Geometry: see drawing. Coordinates: mm, zero at the bounding-box minimum. Round coordinates to 2 decimals unless told otherwise and drop trailing zeros. Order: outer loops, then holes, each group sorted by start corner. A loop starts at its lowest first (then second) coordinate and runs counter-clockwise, first axis right, second up. Notation, with made-up numbers: (76, 50.5) -> (82, 50.5) arc R22 ccw to (82, 73.5) -> close; hole circle Ø4 at (8, 51.5). An arc over 180 degrees is marked (long way). Put each result on its own line as item: value.
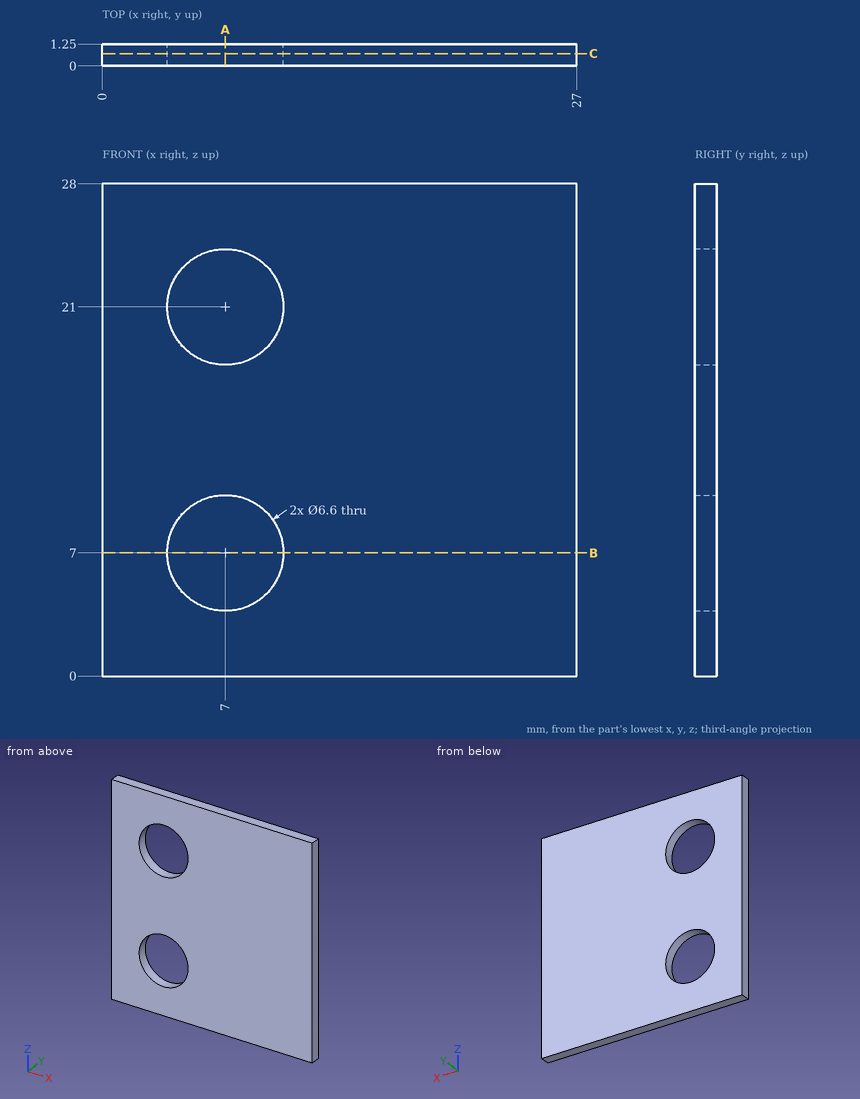
1. Cut plane A-A on x = 7. Return loops of the section in (y, z), and give its area (3 significant figures).
Ans:
outline: (0, 0) -> (1.25, 0) -> (1.25, 3.7) -> (0, 3.7) -> close; (0, 10.3) -> (1.25, 10.3) -> (1.25, 17.7) -> (0, 17.7) -> close; (0, 24.3) -> (1.25, 24.3) -> (1.25, 28) -> (0, 28) -> close
area: 18.5 mm²
2. Cut plane C-C on y = 0.7. Return loops of the section in (x, z).
Ans:
outline: (0, 0) -> (27, 0) -> (27, 28) -> (0, 28) -> close; hole circle Ø6.6 at (7, 7); hole circle Ø6.6 at (7, 21)
3. Cut plane B-B on z = 7. Return loops of the section in (x, y).
Ans:
outline: (0, 0) -> (3.7, 0) -> (3.7, 1.25) -> (0, 1.25) -> close; (10.3, 0) -> (27, 0) -> (27, 1.25) -> (10.3, 1.25) -> close
4. Material intervals for probe 1 along Z at (x, y) = (7, 0.5); probe 2 along X at (y, z) = (0.9, 7); probe 3 along X at (y, z) = (0.95, 5.25), sorted ascending.
Ans:
probe 1: 0 to 3.7, 10.3 to 17.7, 24.3 to 28
probe 2: 0 to 3.7, 10.3 to 27
probe 3: 0 to 4.2, 9.8 to 27
